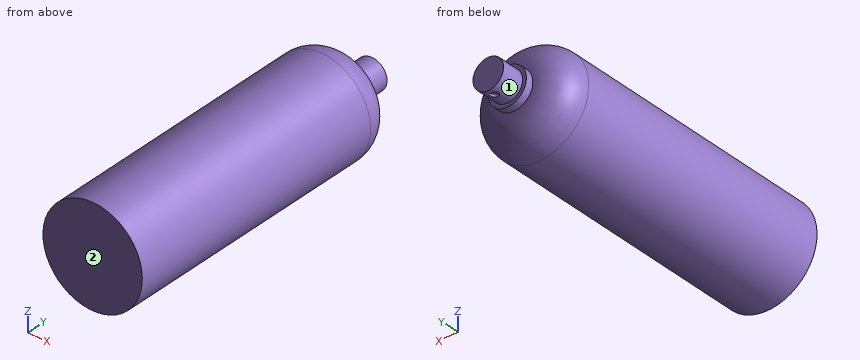
```python
from build123d import *

# Parameters (mm, degrees)
SKETCH_1_R          = 32.5
EXTRUDE_1_DEPTH     = 200
FILLET_1_R          = 20
SKETCH_2_R          = 10
EXTRUDE_2_DEPTH     = 20
CUT_EXTRUDE_START   = -10
SKETCH_3_R          = 2.5
CUT_EXTRUDE_1_DEPTH = 2
SKETCH_2_3_R        = 12.5
SKETCH_2_3_R_2      = 10
EXTRUDE_3_DEPTH     = 5


with BuildPart() as part:
    # Sketch 1 → Extrude 1 (new body)
    with BuildSketch(Plane(origin=(0, 0, 0), x_dir=(1, 0, 0), z_dir=(0, 1, 0))):
        with Locations(Location((0, 0, 0), (0, 0, 270))):
            Circle(SKETCH_1_R)
    extrude(amount=EXTRUDE_1_DEPTH)

    # Fillet 1
    fillet_1_edges = [part.edges().sort_by_distance(p)[0] for p in [
        (0, 200, -32.5),
    ]]
    fillet(fillet_1_edges, radius=FILLET_1_R)

    # Sketch 2 → Extrude 2 (add)
    with BuildSketch(Plane(origin=(0, 200, 0), x_dir=(1, 0, 0), z_dir=(0, 1, 0))):
        with Locations(Location((0, 0, 0), (0, 0, 270))):
            Circle(SKETCH_2_R)
    extrude(amount=EXTRUDE_2_DEPTH)

    # Sketch 3 → Cut-Extrude 1 (cut)
    with BuildSketch(Plane.XY.offset(CUT_EXTRUDE_START)):
        with Locations(Location((0, 215, 0), (0, 0, 90))):
            Circle(SKETCH_3_R)
    extrude(amount=CUT_EXTRUDE_1_DEPTH, mode=Mode.SUBTRACT)

    # Sketch 2_3 → Extrude 3 (add)
    with BuildSketch(Plane(origin=(0, 200, 0), x_dir=(1, 0, 0), z_dir=(0, 1, 0))):
        with Locations(Location((0, 0, 0), (0, 0, 270))):
            Circle(SKETCH_2_3_R)
        with Locations(Location((0, 0, 0), (0, 0, 270))):
            Circle(SKETCH_2_3_R_2, mode=Mode.SUBTRACT)
    extrude(amount=EXTRUDE_3_DEPTH)


solid = part.part
```
Read the model definition and answer for the solid it produces. Units are mm, in the model's axes. Face numbers are marked on the shaded views. A direction names the side the tool comes from. Coordinates: 2 decimals unless noted, no trailing zeros. Loops run counter-clockwise (first coordinate to the right, second up) from the corner with the lowest first, then second, coordinate; pieces in that order, holes last. Notation, with made-up numbers: (-29, 12) - (7, 12) arc R18 cw to (7, 17) - close; hole circle Ø4 at (40, -13.75). An arc over 180 degrees is marked (long way). Answer in a Markdown table with one row per item.
1. Straight lines are drawn through the part: line 1 (X direction, y = 215, z = -9.15); line 2 (X direction, y = 215, z = -8.95); line 3 (Z direction, x = 10.5, y = 191). For each, find the intervals that lie inside material, in ascending order.
Conclusion:
| item | result |
|---|---|
| line 1 | x = -4.03 to -2.5, 2.5 to 4.03 |
| line 2 | x = -4.46 to -2.5, 2.5 to 4.46 |
| line 3 | z = -27.25 to 27.25 |
2. Given pin 1 (1.5 mm diameter, centred on x = -1, y = 215.5, fed in from -Z); pin 2 (12 mm diameter, centred on y = 129.5, z = -4.5, fed in from -X); pin 3 (5 mm diameter, centred on x = -4, z = 12.5, fed in from +Y), each flat-ended and moving along its own axis, determine where each tip first touches the part or whether it passes through.
Conclusion:
| item | result |
|---|---|
| pin 1 | stops at z = -8 |
| pin 2 | stops at x = -32.5 |
| pin 3 | stops at y = 205 |
3. Which of the six approach directions +Z, -Z, +X, -X, +Y, -Y give full straight-line access (tool end or side, diameter ignored) to the marked faces 1 and 2?
Conclusion:
| item | result |
|---|---|
| face 1 | +Y |
| face 2 | +Z, -Z, +X, -X, -Y |
4. Find section B-B, the plane y = 215. Write down the section's boundary in (x, z), then the cut area to 3 significant figures.
Conclusion:
| item | result |
|---|---|
| outline | (-2.5, -9.68) - (-2.5, -8) - (2.5, -8) - (2.5, -9.68) arc R10 ccw (long way) to start |
| area | 305 mm² |
5. Find section A-A, the plane y = 163. Write down the section's boundary in (x, z).
Conclusion:
| item | result |
|---|---|
| outline | circle Ø65 at (0, 0) |
